Autodesk Inventor part; units mm, degrees
ref_plane "YZ Plane" through (0, 0, 0) normal (1, 0, 0) x (0, 1, 0)
ref_plane "XZ Plane" through (0, 0, 0) normal (0, 1, 0) x (-1, 0, 0)
ref_plane "XY Plane" through (0, 0, 0) normal (0, 0, 1) x (1, 0, 0)
sketch "Sketch2" plane through (0, 0, 0) normal (0, 1, 0) x (-1, 0, 0)
  line L0 (19.2111, 42.6505) -> (-8.7889, 42.6505)
  line L1 (-8.7889, 42.6505) -> (-8.7889, -32.8495)
  line L2 (-8.7889, -32.8495) -> (19.2111, -32.8495)
  line L3 (19.2111, -32.8495) -> (19.2111, 42.6505)
  dimension "d11" = 75.5
  dimension "d41" = 28
extrude "Extrusion3" add sketch "Sketch2" along normal blind 3
sketch "Sketch6" plane through (0, 3, 0) normal (0, 1, 0) x (1, 0, 0)
  line L0 (-16.2111, -12.0368) -> (-2.2111, -12.0368)
  line L1 (-2.2111, -12.0368) -> (-2.2111, 1.9632)
  line L2 (-2.2111, 1.9632) -> (-16.2111, 1.9632)
  line L3 (-16.2111, 1.9632) -> (-16.2111, -12.0368)
  line L4 (-6.3559, -35.9231) -> (5.8695, -29.1012)
  line L5 (5.8695, -29.1012) -> (-0.9523, -16.8758)
  line L6 (-0.9523, -16.8758) -> (-13.1778, -23.6976)
  line L7 (-13.1778, -23.6976) -> (-6.3559, -35.9231)
  line L8 (-0.9523, 6.8022) -> (5.8695, 19.0276)
  line L9 (5.8695, 19.0276) -> (-6.3559, 25.8495)
  line L10 (-6.3559, 25.8495) -> (-13.1778, 13.6241)
  line L11 (-13.1778, 13.6241) -> (-0.9523, 6.8022)
  circle A0 centre (34.6298, -5.0368) radius 37.5 construction
  line L12 (-19.2111, 32.8495) -> (-19.2111, -42.6505)
  line L13 (8.7889, 32.8495) -> (-19.2111, 32.8495)
  point P0 (0, 0)
  dimension "d30" = 75
  dimension "d31" = 14
  dimension "d32" = 14
  dimension "d33" = 14
  dimension "d34" = 14
  dimension "d35" = 14
  dimension "d36" = 14
  dimension "d37" = 5
  dimension "d38" = 5
  dimension "d39" = 3
  dimension "d40" = 7
extrude "Extrusion4" cut sketch "Sketch6" against normal through all
properties part number "k2_t_top"
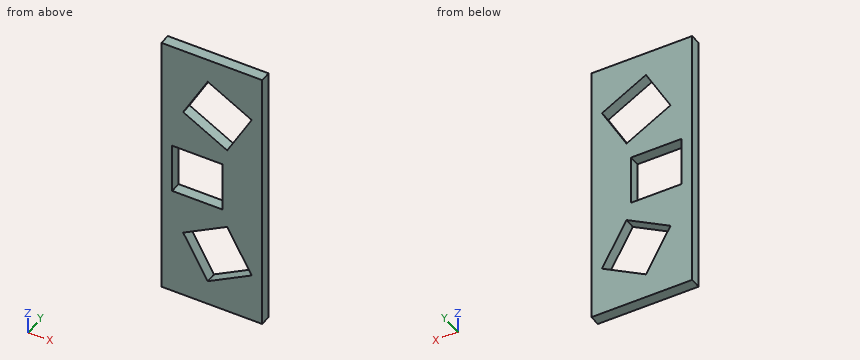
Input: part model. Units: mm. Frame: model coordinates. Round coordinates to 2 decimals unless told otherwise and drop trailing zeros. Order: outer loops, then holes, each group sorted by start corner. A loop starts at its lowest first (then second) coordinate and runs counter-clockwise, first axis right, second up. Notation, with made-up numbers: (72, -30.75) - (115, -30.75) arc R10 cw to (115, -16.75) - close; hole circle Ø4 at (1, -10.75). An arc over 180 degrees is marked (long way). Use a Markdown table: item, result.
1. Section C-C on z = -12.5. Return the cut outline in (x, y).
Evaluation:
| item | result |
|---|---|
| outline | (-19.21, 0) - (-11.16, 0) - (-11.16, 3) - (-19.21, 3) - close; (2.23, 0) - (8.79, 0) - (8.79, 3) - (2.23, 3) - close |
2. Section A-A on y = 1.8. Return the cut outline in (x, z), then the cut area to 3 significant figures.
Evaluation:
| item | result |
|---|---|
| outline | (-19.21, -32.85) - (8.79, -32.85) - (8.79, 42.65) - (-19.21, 42.65) - close; hole (-16.21, -1.96) - (-2.21, -1.96) - (-2.21, 12.04) - (-16.21, 12.04) - close; hole (-13.18, -13.62) - (-6.36, -25.85) - (5.87, -19.03) - (-0.95, -6.8) - close; hole (-13.18, 23.7) - (-0.95, 16.88) - (5.87, 29.1) - (-6.36, 35.92) - close |
| area | 1,530 mm^2 |
3. Material intervals for probe 1 along Z at (x, y) = (-5.25, 1.1); probe 2 along Z at (x, y) = (-7, 0.7); probe 3 along X at (y, z) = (2.05, 5), sorted ascending.
Evaluation:
| item | result |
|---|---|
| probe 1 | -32.85 to -25.23, -9.2 to -1.96, 12.04 to 19.27, 35.31 to 42.65 |
| probe 2 | -32.85 to -24.7, -10.18 to -1.96, 12.04 to 20.25, 34.77 to 42.65 |
| probe 3 | -19.21 to -16.21, -2.21 to 8.79 |
4. Section B-B on x = -10.25. Return the cut outline in (y, z).
Evaluation:
| item | result |
|---|---|
| outline | (0, -32.85) - (3, -32.85) - (3, -18.87) - (0, -18.87) - close; (0, -11.99) - (3, -11.99) - (3, -1.96) - (0, -1.96) - close; (0, 12.04) - (3, 12.04) - (3, 22.06) - (0, 22.06) - close; (0, 28.94) - (3, 28.94) - (3, 42.65) - (0, 42.65) - close |
5. First-contact query: pin 1 (4 mm diameter, centred on x = -14.5, z = 11, fed in from -Y). Flat tip, straight axial feed; report the tip coordinate or a pass-through.
Evaluation:
| item | result |
|---|---|
| pin 1 | y = 0 |
6. Section D-D on x = 3.5. Return the cut outline in (y, z).
Evaluation:
| item | result |
|---|---|
| outline | (0, -32.85) - (3, -32.85) - (3, -20.35) - (0, -20.35) - close; (0, -14.78) - (3, -14.78) - (3, 24.85) - (0, 24.85) - close; (0, 30.42) - (3, 30.42) - (3, 42.65) - (0, 42.65) - close |
